```python
from build123d import *

# Parameters (mm, degrees)
PAD_DEPTH       = 1.5
PAD001_DEPTH    = 27
PAD002_DEPTH    = 11
SKETCH003_W     = 10
SKETCH003_H     = 2
POCKET_DEPTH    = 16
SKETCH004_W     = 8
SKETCH004_H     = 2
POCKET001_DEPTH = 4
SKETCH005_R     = 4
POCKET002_DEPTH = 2
SKETCH006_R     = 5
POCKET003_DEPTH = 27
PAD003_DEPTH    = 27
PAD004_DEPTH    = 1.5
SKETCH009_R     = 1
POCKET004_DEPTH = 5
SKETCH010_R     = 1
POCKET005_DEPTH = 5


with BuildPart() as obj1:
    # Sketch → Pad (new body)
    with BuildSketch(Plane.XY):
        Polygon((-20, 11.5), (23, 11.5), (23, 0), (10, 0), (6.5, -16), (-6.5, -16), (-10, 0), (-20, 0), align=None)
    extrude(amount=PAD_DEPTH)

    # Sketch001 → Pad001 (new body)
    with BuildSketch(Plane.XY.offset(1.5)):
        Polygon((-20, 0), (-20, 1.5), (-8.890625, 1.5), (-5.5, -14), (5.5, -14), (8.890625, 1.5), (23, 1.5), (23, 0), (10, 0), (6.5, -16), (-6.5, -16), (-10, 0), align=None)
    extrude(amount=PAD001_DEPTH)

    # Sketch002 → Pad002 (new body)
    with BuildSketch(Plane.XY.offset(1.5)):
        Polygon((-6.15625, -11), (-4, -11), (-4, -9.5), (-6.484375, -9.5), align=None)
        Polygon((6.484375, -9.5), (4, -9.5), (4, -11), (6.15625, -11), align=None)
    extrude(amount=PAD002_DEPTH)

    # Sketch003 → Pocket (cut)
    with BuildSketch(Plane.XY.offset(28.5)):
        with Locations((0, -15)):
            Rectangle(SKETCH003_W, SKETCH003_H)
    extrude(amount=-POCKET_DEPTH, mode=Mode.SUBTRACT)

    # Sketch004 → Pocket001 (cut)
    with BuildSketch(Plane.XY.offset(12.5)):
        with Locations((0, -15)):
            Rectangle(SKETCH004_W, SKETCH004_H)
    extrude(amount=-POCKET001_DEPTH, mode=Mode.SUBTRACT)

    # Sketch005 → Pocket002 (cut)
    with BuildSketch(Plane.XZ.offset(16)):
        with Locations((0, 8.5)):
            Circle(SKETCH005_R)
    extrude(amount=-POCKET002_DEPTH, mode=Mode.SUBTRACT)

    # Sketch006 → Pocket003 (cut)
    with BuildSketch(Plane.XY.offset(28.5)):
        with Locations((7.390625, 2.5)):
            Circle(SKETCH006_R)
    extrude(amount=-POCKET003_DEPTH, mode=Mode.SUBTRACT)

    # Sketch007 → Pad003 (new body)
    with BuildSketch(Plane.XY.offset(1.5)):
        with BuildLine():
            ThreePointArc((9.179934789, -3.7488695361), (11.7128746974, -2.3547046824), (13.390625, 0))
            Line((11.7207520189, 0), (13.390625, 0))
            ThreePointArc((9.5616048305, -2.0040922033), (10.792123781, -1.1646699774), (11.7207520189, 0))
            Line((9.5616048305, -2.0040922033), (9.179934789, -3.7488695361))
        make_face()
    extrude(amount=PAD003_DEPTH)

    # Sketch008 → Pad004 (new body)
    with BuildSketch(Plane(origin=(0, 0, 1.5), x_dir=(1, 0, 0), z_dir=(0, 0, -1))):
        with BuildLine():
            ThreePointArc((13.390625, 0), (11.7128746974, 2.3547046824), (9.179934789, 3.7488695361))
            Line((9.179934789, 3.7488695361), (10, 0))
            Line((10, 0), (13.390625, 0))
        make_face()
    extrude(amount=PAD004_DEPTH)

    # Sketch009 → Pocket004 (cut)
    with BuildSketch(Plane.XZ):
        with Locations((-15, 20.5)):
            Circle(SKETCH009_R)
        with Locations((18.1953125, 20.5)):
            Circle(SKETCH009_R)
    extrude(amount=-POCKET004_DEPTH, mode=Mode.SUBTRACT)

    # Sketch010 → Pocket005 (cut)
    with BuildSketch(Plane(origin=(0, 0, 0), x_dir=(1, 0, 0), z_dir=(0, 0, -1))):
        with Locations((-15, -5.75)):
            Circle(SKETCH010_R)
        with Locations((18.1953125, -5.75)):
            Circle(SKETCH010_R)
    extrude(amount=-POCKET005_DEPTH, mode=Mode.SUBTRACT)


with BuildPart() as obj2:
    # Part__Mirroring: instance of obj1
    add(obj1.part.mirror(Plane(origin=(0, 0, 0), x_dir=(0, -1, 0), z_dir=(1, 0, 0))))


solid = obj2.part
```
Verification items for the finished model (mm, model axes). A direction names the side the tool comes from. Give positions to 0.01 mm unless a question says otherwise; leave off trailing zeros. Write each loop counter-clockwise with the first axis right and the second up, starting at its lowest first coordinate (ties: lowest second). Pieces come first, ordered by that corner, then holes. Notation, with made-up numbers: (67, 12) - (97, 12) arc R15 ccw to (97, 37) - close; hole circle Ø2 at (-23, 83.5). An arc over 180 degrees is marked (long way). Put each result on its own line as item: value.
Q1. Set-up check for faces 5 (the face through (-5, -9.5, 7)), 6 (the face through (15, 0, 14)), 7 (the face through (4.5, -15, 12.5)), 8 (the face through (14.54, 0.74, 19.61)), 9 (the face through (15, 1.5, 15)): record each of +Z, -Z, +X, -X, +Y, -Y from which the full face is reachable in a straight line by a thin tool's end or side.
Result:
face 5: +Z, +Y
face 6: +Z, -Z, +X, -Y
face 7: +Z, +Y, -Y
face 8: +Y, -Y
face 9: +Z, +X, -X, +Y
Q2. Section check A-A on z = 20.5. Record the cut outline in (x, y).
Result:
outline: (-23, 0) - (-19.2, 0) - (-19.2, 1.5) - (-23, 1.5) - close; (-17.2, 0) - (-13.39, 0) arc R6.5 ccw to (-9.18, -3.75) - (-6.5, -16) - (-5, -16) - (-5, -14) - (-5.5, -14) - (-8.02, -2.46) arc R5 cw to (-12.29, 1.5) - (-17.2, 1.5) - close; (5, -16) - (6.5, -16) - (10, 0) - (14, 0) - (14, 1.5) - (8.89, 1.5) - (5.5, -14) - (5, -14) - close; (16, 0) - (20, 0) - (20, 1.5) - (16, 1.5) - close
Q3. Section check D-D on x = 0. Record the cut outline in (y, z), and give its area (4 significant figures).
Result:
outline: (-16, 0) - (11.5, 0) - (11.5, 1.5) - (-14, 1.5) - (-14, 4.5) - (-16, 4.5) - close
area: 47.25 mm2
Q4. Mould release check, pull along X, two halves, no side actions. Record for faces 1 (the face through (4, -10, 7)), 2 (the face through (-1, 11.5, 1)), 3 (the face through (20, 1, 12)), 4 (the face through (7.22, -6.14, 14.81)): released by +X, released by -X, zero draft, split by the parting line, or undercut.
Result:
face 1: undercut
face 2: zero draft
face 3: released by +X
face 4: undercut
Q5. Scan lines: probe 1 along X at (y, z) = (5.75, 0.75); probe 2 along Z at (x, y) = (15, 0.7); probe 3 along Y at (x, z) = (15, 0.3). Record each from-to range of solid material in increasing order. Write a range as from..to.
Result:
probe 1: -23..-19.2, -17.2..14, 16..20
probe 2: 0..19.5, 21.5..28.5
probe 3: 0..4.75, 6.75..11.5
Q6. Depth check by flat-ended pin: P1, Ø0.8, axis at y = -10, z = 7.5, coming from the +X side; P2, Ø2.5, axis at x = -18.2, z = 20.5, coming from the +Y side; P3, Ø12, axis at x = 9, y = 4.5, coming from the -Z side; P4, Ø1, axis at y = -15, z = 10.5, coming from the +X side. Enter the tip coordinate at first touch or a pass-through.
Result:
P1: x = 7.9
P2: y = 1.5
P3: z = 0
P4: x = 6.83
Q7. Section check B-B on x = 15. Record the cut outline in (y, z).
Result:
outline: (0, 0) - (4.75, 0) - (4.75, 1.5) - (1.5, 1.5) - (1.5, 19.5) - (0, 19.5) - close; (0, 21.5) - (1.5, 21.5) - (1.5, 28.5) - (0, 28.5) - close; (6.75, 0) - (11.5, 0) - (11.5, 1.5) - (6.75, 1.5) - close
Q8. Section check C-C on z = 17.5. Record the cut outline in (x, y).
Result:
outline: (-23, 0) - (-13.39, 0) arc R6.5 ccw to (-9.18, -3.75) - (-6.5, -16) - (-5, -16) - (-5, -14) - (-5.5, -14) - (-8.02, -2.46) arc R5 cw to (-12.29, 1.5) - (-23, 1.5) - close; (5, -16) - (6.5, -16) - (10, 0) - (20, 0) - (20, 1.5) - (8.89, 1.5) - (5.5, -14) - (5, -14) - close
